Autodesk Fusion 360 part; units mm, degrees
sketch "Top" plane through (0, 0, 0) normal (0, 0, 1) x (1, 0, 0)
  line L0 (59.2894, -12.484) -> (59.2841, -12.484)
  line L1 (59.2841, -12.484) -> (59.2841, -12.4898)
  line L2 (59.2841, -12.4898) -> (51.2779, -12.4898)
  line L3 (51.2779, -12.4898) -> (51.2779, -14.4245)
  line L4 (51.2779, -14.4245) -> (50.2771, -14.4245)
  line L5 (50.2771, -14.4245) -> (50.2771, -11.4736)
  line L6 (50.2771, -11.4736) -> (50.4315, -11.4736)
  line L7 (50.4315, -11.4736) -> (50.4315, -11.4723)
  line L8 (50.4315, -11.4723) -> (58.2887, -11.5)
  line L9 (58.2887, -11.5) -> (58.283, -10.5632)
  line L10 (58.283, -10.5632) -> (50.2771, -10.5355)
  line L11 (50.2771, -10.5355) -> (50.2828, -9.5486)
  line L12 (50.2828, -9.5486) -> (59.2837, -9.5486)
  line L13 (59.2837, -9.5486) -> (59.2837, -9.565)
  line L14 (59.2837, -9.565) -> (59.2894, -9.565)
  line L15 (59.2894, -9.565) -> (59.2894, -12.484)
  line L16 (49.1011, -10.5494) -> (44.8406, -10.5786)
  line L17 (44.8406, -10.5786) -> (44.8406, -14.4537)
  line L18 (44.8406, -14.4537) -> (39.5795, -14.4245)
  line L19 (39.5795, -14.4245) -> (39.5795, -13.4237)
  line L20 (39.5795, -13.4237) -> (43.8385, -13.4237)
  line L21 (43.8385, -13.4237) -> (43.8413, -9.5486)
  line L22 (43.8413, -9.5486) -> (49.1011, -9.5486)
  line L23 (49.1011, -9.5486) -> (49.1011, -10.5494)
  line L24 (31.7113, -12.5044) -> (31.7113, -14.4245)
  line L25 (31.7113, -14.4245) -> (30.7106, -14.4245)
  line L26 (30.7106, -14.4245) -> (30.7106, -11.5015)
  line L27 (30.7106, -11.5015) -> (30.8648, -11.5015)
  line L28 (30.8648, -11.5015) -> (30.8648, -11.5001)
  line L29 (30.8648, -11.5001) -> (38.7247, -11.4943)
  line L30 (38.7247, -11.4943) -> (38.7192, -10.5436)
  line L31 (38.7192, -10.5436) -> (30.7106, -10.5494)
  line L32 (30.7106, -10.5494) -> (30.7161, -9.5486)
  line L33 (30.7161, -9.5486) -> (39.7172, -9.5486)
  line L34 (39.7172, -9.5486) -> (39.7172, -9.565)
  line L35 (39.7172, -9.565) -> (39.7227, -9.565)
  line L36 (39.7227, -9.565) -> (39.7227, -12.4987)
  line L37 (39.7227, -12.4987) -> (39.7172, -12.4987)
  line L38 (39.7172, -12.4987) -> (39.7172, -12.5044)
  line L39 (39.7172, -12.5044) -> (31.7113, -12.5044)
  line L40 (64, -3) -> (64, 0)
  line L41 (64, 0) -> (26, 0)
  line L42 (26, 0) -> (26, -3)
  line L43 (26, -3) -> (0, -79)
  line L44 (0, -79) -> (0, -82)
  line L45 (0, -82) -> (16, -82)
  line L46 (16, -82) -> (35.8941, -36.045)
  spline S0 degree 3 poles (35.8941, -36.045) (39.3461, -28.0709) (50.6539, -28.0709) (54.106, -36.045) knots 7 7 7 7 8 8 8 8
  line L47 (54.106, -36.045) -> (74, -82)
  line L48 (74, -82) -> (90, -82)
  line L49 (90, -82) -> (90, -79)
  line L50 (90, -79) -> (64, -3)
extrude "Extrude1" add sketch "Top" along normal blind 32.47
sketch "Side" plane through (0, 0, 0) normal (1, 0, 0) x (0, 1, 0)
  line L0 (-82, 37.505) -> (-82, 32.4661)
  line L1 (-82, 32.4661) -> (-74, 32.4661)
  line L2 (-74, 32.4661) -> (-74, 29.4661)
  line L3 (-74, 29.4661) -> (-79, 29.4661)
  line L4 (-79, 29.4661) -> (-79, 2.9661)
  line L5 (-79, 2.9661) -> (-3, 2.9661)
  line L6 (-3, 2.9661) -> (-3, 25.9661)
  spline S0 degree 3 poles (-3, 25.9661) (-3.8284, 25.9661) (-4.5, 26.6377) (-4.5, 27.4661) (-4.5, 28.2945) (-3.8284, 28.9661) (-3, 28.9661) knots 7 7 7 7 8 8 8 9 9 9 9
  line L7 (-3, 28.9661) -> (0, 28.9661)
  line L8 (0, 28.9661) -> (0, 37.505)
  line L9 (0, 37.505) -> (-82, 37.505)
extrude "Extrude2" cut sketch "Side" along normal blind 90
hole "Hole1" at (29.5044, -23.6505, 2.9661) direction (0, 0, -1) diameter 3.5 depth 3 tip angle 118 countersink diameter 5.5 countersink angle 90
hole "Hole2" at (60.4957, -23.6505, 2.9661) direction (0, 0, -1) diameter 3.5 depth 3 tip angle 118 countersink diameter 5.5 countersink angle 90
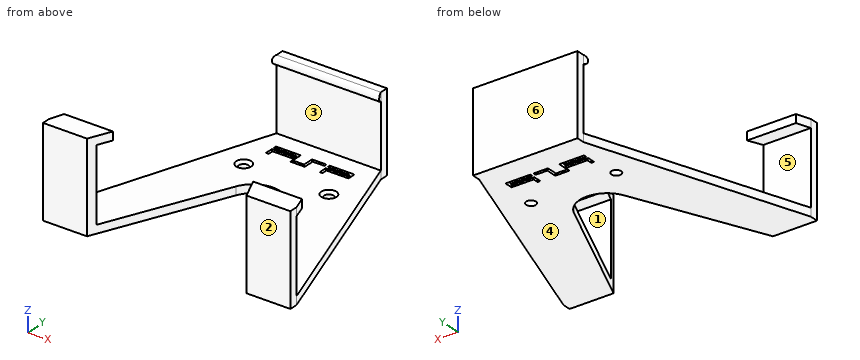
Input: part model. Units: mm. Frame: model coordinates. Face numbers are marked on the shaded views. A direction names the side the tool comes from. Give positions to 0.01 mm unless a question says otherwise; leave off trailing zeros. Order: outer loops, then holes, each group sorted by start corner. A loop starts at its lowest first (then second) coordinate and runs counter-clockwise, first axis right, second up.
1. Set-up query: the marked faces 1, 2 and 3. Return all of +Z, -Z, +X, -X, +Y, -Y with unobstructed straight access to the full face (end or side cutting, diameter ignored); none if empty.
Computed:
face 1: +X, -X, +Y
face 2: +Z, -Z, +X, -X, -Y
face 3: +X, -X, -Y
2. Line query: probe 1 along Y at (x, z) = (11.5, 20.5); probe 2 along Y at (x, z) = (59, 5.5); probe 3 along Z at (x, y) = (85.5, -68). Output: solid intervals per line, ascending.
Computed:
probe 1: y = -82 to -79
probe 2: y = -3 to 0
probe 3: z = 0 to 2.97
3. Cut plane B-B (y = -61). Return loops of the section in (x, z), and give its area (3 significant figures).
Computed:
outline: (6.16, 0) - (25.09, 0) - (25.09, 2.97) - (6.16, 2.97) - close; (64.91, 0) - (83.84, 0) - (83.84, 2.97) - (64.91, 2.97) - close
area: 112 mm2
4. Pin query (flat end, axial travel): pin 1 Ø8 at (x, z) = (16, 12.5) entering from +Y; pin 2 Ø3.5 at (x, z) = (41, 2) entering from -Y; pin 3 Ø0.5 at (y, z) = (-14, 2) entering from +X; pin 4 Ø6 at (y, z) = (-40.5, 8.5) entering from -X. Return the tip coordinate at first contact, or that it passes through.
Computed:
pin 1: stops at y = -79
pin 2: stops at y = -31.87
pin 3: stops at x = 67.85
pin 4: passes through
5. Cut plane A-A (z = 20). Return loops of the section in (x, y), and give its area (3 significant figures).
Computed:
outline: (0, -82) - (16, -82) - (17.3, -79) - (0, -79) - close; (26, -3) - (64, -3) - (64, 0) - (26, 0) - close; (72.7, -79) - (74, -82) - (90, -82) - (90, -79) - close
area: 214 mm2
6. Cut plane C-C (x = 83). Return loops of the section in (y, z), and give its area (3 significant figures).
Computed:
outline: (-82, 0) - (-58.54, 0) - (-58.54, 2.97) - (-79, 2.97) - (-79, 29.47) - (-74, 29.47) - (-74, 32.47) - (-82, 32.47) - close
area: 173 mm2
7. Draft query along Z for the marked faces 4, 5 and 6. Return one class per face: released by +Z, released by -Z, zero draft, split by the parting line, or undercut.
Computed:
face 4: released by -Z
face 5: undercut
face 6: zero draft
8. Cut plane D-D (y = -39). Return loops of the section in (x, z), and give its area (3 significant figures).
Computed:
outline: (13.68, 0) - (34.61, 0) - (34.61, 2.97) - (13.68, 2.97) - close; (55.39, 0) - (76.32, 0) - (76.32, 2.97) - (55.39, 2.97) - close
area: 124 mm2
